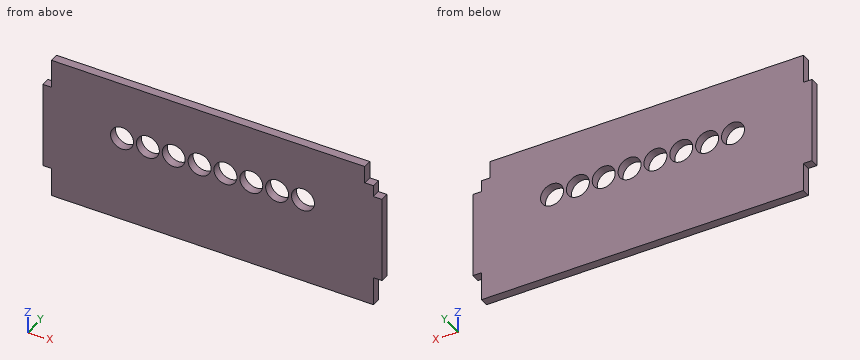
```python
from build123d import *

# Parameters (mm, degrees)
LED_1_OUTLINE_R     = 2.25
LED_1_DEPTH         = 3
SKETCH_1_R          = 4
CUT_EXTRUDE_1_DEPTH = 3


# Read off the part's stored shape, not the designer's step: 基体零件-LED板-1
with BuildPart() as part:
    # 基体零件-LED板-1 outline → 基体零件-LED板-1 (new body)
    with BuildSketch(Plane(origin=(0, 0, 0), x_dir=(1, 0, 0), z_dir=(0, 1, 0))):
        Polygon((-3, -140), (0, -140), (0, -110), (-3, -110), (-3, -100), (-115, -100), (-115, -110), (-118, -110), (-118, -140), (-115, -140), (-115, -150), (-6.001970153, -150), (-6.001970153, -144), (-3, -144), align=None)
        with Locations((-90.5, -130)):
            Circle(LED_1_OUTLINE_R, mode=Mode.SUBTRACT)
        with Locations((-81.5, -130)):
            Circle(LED_1_OUTLINE_R, mode=Mode.SUBTRACT)
        with Locations((-72.5, -130)):
            Circle(LED_1_OUTLINE_R, mode=Mode.SUBTRACT)
        with Locations((-63.5, -130)):
            Circle(LED_1_OUTLINE_R, mode=Mode.SUBTRACT)
        with Locations((-54.5, -130)):
            Circle(LED_1_OUTLINE_R, mode=Mode.SUBTRACT)
        with Locations((-45.5, -130)):
            Circle(LED_1_OUTLINE_R, mode=Mode.SUBTRACT)
        with Locations((-36.5, -130)):
            Circle(LED_1_OUTLINE_R, mode=Mode.SUBTRACT)
        with Locations((-27.5, -130)):
            Circle(LED_1_OUTLINE_R, mode=Mode.SUBTRACT)
    extrude(amount=LED_1_DEPTH)

    # 草图1 → 切除-拉伸1 (cut)
    with BuildSketch(Plane(origin=(0, 3, 0), x_dir=(1, 0, 0), z_dir=(0, 1, 0))):
        with Locations(Location((-90.5, -130, 0), (0, 0, 270))):
            Circle(SKETCH_1_R)
        with Locations(Location((-81.5, -130, 0), (0, 0, 270))):
            Circle(SKETCH_1_R)
        with Locations(Location((-72.5, -130, 0), (0, 0, 270))):
            Circle(SKETCH_1_R)
        with Locations(Location((-63.5, -130, 0), (0, 0, 270))):
            Circle(SKETCH_1_R)
        with Locations(Location((-54.5, -130, 0), (0, 0, 270))):
            Circle(SKETCH_1_R)
        with Locations(Location((-45.5, -130, 0), (0, 0, 270))):
            Circle(SKETCH_1_R)
        with Locations(Location((-36.5, -130, 0), (0, 0, 270))):
            Circle(SKETCH_1_R)
        with Locations(Location((-27.5, -130, 0), (0, 0, 270))):
            Circle(SKETCH_1_R)
    extrude(amount=-CUT_EXTRUDE_1_DEPTH, mode=Mode.SUBTRACT)


solid = part.part
```
Can you work these out from the model? Positions are in its coordinate system, mm. Give positions to 0.01 mm unless a question says otherwise; leave off trailing zeros. Loops run counter-clockwise (first coordinate to the right, second up) from the corner with the lowest first, then second, coordinate; pieces in that order, holes last. Notation, with made-up numbers: M 53,-37.75 L 102,-37.75 A29 cw 102,-5.75 Z; hole C 30,55.25 d1. An arc over 180 degrees is marked long. One line per question, with ' | ' between items. Start each with the question number.
Q1. If we section it at C-C (z = 142.5): Please give me the cut outline in (x, y).
Q2. If we section it at B-B (y = 1.2): State how many separate pieces and enclosed holes the cut face has, plus the area to 3 significant figures.
Q3. If I drill on line 1 (X direction, y = 2.5, z = 146); line 2 (X direction, y = 0.65, z = 105.5); line 3 (Z direction, x = -40, y = 2.15), over which ranges is the centre line in solid material (lowest first)? Write a range as from..to.
Q4. If we section it at A-A (x = -36.5): Please give me the cut outline in (y, z), plus the area to 3 significant figures.
Q5. For pin 1 Ø1.5 at (y, z) = (2, 141.5) entering from +X; pin 2 Ø1.5 at (x, y) = (-1, 2) entering from -Z; pin 3 Ø0.9 at (y, z) = (1.5, 144) entering from -X, each with a flat end and sliding along its axis, tell me the tip position at first contact or that it passes through.
Q6. If we section it at D-D (x = -92.5): Please give me the cut outline in (y, z), plus the area to 3 significant figures.
Computed:
1) outline: M -115,0 L -3,0 L -3,3 L -115,3 Z
2) separate pieces: 1 | enclosed holes: 8 | area: 5,360 mm²
3) line 1: x = -115..-6 | line 2: x = -115..-3 | line 3: z = 100..128.06, 131.94..150
4) outline: M 0,100 L 3,100 L 3,126 L 0,126 Z; M 0,134 L 3,134 L 3,150 L 0,150 Z | area: 126 mm²
5) pin 1: stops at x = -3 | pin 2: stops at z = 110 | pin 3: stops at x = -115
6) outline: M 0,100 L 3,100 L 3,126.54 L 0,126.54 Z; M 0,133.46 L 3,133.46 L 3,150 L 0,150 Z | area: 129 mm²
